```python
from build123d import *

# Parameters (mm, degrees)
SKETCH_W               = 20
SKETCH_H               = 7
PAD_DEPTH              = 7
FILLET_R               = 6.5
MIRROR_ROLL_ANGLE      = -179.860318
MIRROR_PITCH_ANGLE     = 1.669328
MIRROR_PLACEMENT_ANGLE = 0.337481


with BuildPart() as body:
    # Sketch → Pad (new body)
    with BuildSketch(Plane.XY):
        Polygon((0, 290), (50, 290), (150, 0), (120, 0), (120, 13.2), (30, 13.2), (30, 0), (0, 0), align=None)
        Polygon((15, 210), (15, 130), (89.30566, 130), (61.719453, 210), align=None, mode=Mode.SUBTRACT)
        Polygon((15, 110), (15, 33.2), (122.684971, 33.2), (96.202212, 110), align=None, mode=Mode.SUBTRACT)
        Polygon((18, 280), (18, 230), (54.822902, 230), (37.581522, 280), align=None, mode=Mode.SUBTRACT)
        with Locations((28, 220)):
            Rectangle(SKETCH_W, SKETCH_H, mode=Mode.SUBTRACT)
        with Locations((28, 120)):
            Rectangle(SKETCH_W, SKETCH_H, mode=Mode.SUBTRACT)
        with Locations((70.5, 120)):
            Rectangle(SKETCH_W, SKETCH_H, mode=Mode.SUBTRACT)
        with Locations((28, 23.2)):
            Rectangle(SKETCH_W, SKETCH_H, mode=Mode.SUBTRACT)
        with Locations((111, 23.2)):
            Rectangle(SKETCH_W, SKETCH_H, mode=Mode.SUBTRACT)
    extrude(amount=PAD_DEPTH)

    # Fillet
    fillet_edges = [body.edges().sort_by_distance(p)[0] for p in [
        (0, 0, 3.5),
        (50, 290, 3.5),
        (0, 290, 3.5),
        (150, 0, 3.5),
        (120, 0, 3.5),
        (30, 0, 3.5),
        (61.719453, 210, 3.5),
        (15, 210, 3.5),
        (96.202212, 110, 3.5),
        (15, 110, 3.5),
        (15, 130, 3.5),
        (15, 33.2, 3.5),
        (122.684971, 33.2, 3.5),
        (89.30566, 130, 3.5),
        (30, 13.2, 3.5),
        (120, 13.2, 3.5),
        (18, 280, 3.5),
        (18, 230, 3.5),
        (37.581522, 280, 3.5),
        (54.822902, 230, 3.5),
    ]]
    fillet(fillet_edges, radius=FILLET_R)


with BuildPart() as body_1:
    # Body placement: moved
    add(body.part.moved(Location((-2, 0, 0))))


with BuildPart() as body_mirrored:
    # mirror: instance of Body
    add(body_1.part.mirror(Plane(origin=(159.181488, 124.226166, 5.790833), x_dir=(-0.001618, 0.999999, 0), z_dir=(-0.999887, -0.001617, 0.014919))))


with BuildPart() as body_mirrored_1:
    # mirror roll: moved
    add(body_mirrored.part.rotate(Axis((0, 0, 0), (1, 0, 0)), MIRROR_ROLL_ANGLE))


with BuildPart() as body_mirrored_2:
    # mirror pitch: moved
    add(body_mirrored_1.part.rotate(Axis((0, 0, 0), (0, 1, 0)), MIRROR_PITCH_ANGLE))


with BuildPart() as body_mirrored_3:
    # mirror placement: moved
    add(body_mirrored_2.part.moved(Location((-113.201923, 287.892908, 10.586))).rotate(Axis((-113.201923, 287.892908, 10.586), (0, 0, 1)), MIRROR_PLACEMENT_ANGLE))


solid = body_mirrored_3.part
```
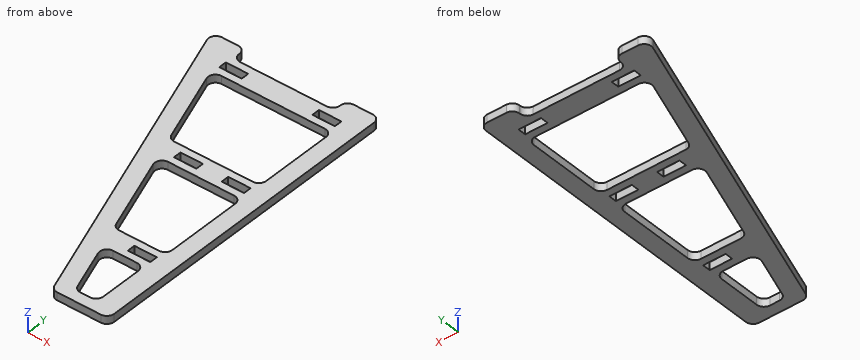
Input: part model. Units: mm. Frame: model coordinates. Give positions to 0.01 mm unless a question says otherwise; leave off trailing zeros. Order: outer loops, then holes, each group sorted by start corner. A loop starts at its lowest first (then second) coordinate and runs counter-clockwise, first axis right, second up.
1. Section B-B on y = 228.5. Return the cut outline in (x, z), and give its area (3 significant figures).
Derived:
outline: (78.31, 5.82) - (78.32, -1.18) - (94.2, -1.17) - (94.19, 5.83) - close; (192.48, -1.1) - (207.48, -1.09) - (207.48, 5.91) - (192.48, 5.9) - close
area: 216 mm2
2. Pin query (flat end, axial travel): pin 1 (1.5 mm diameter, centred on x = 167.5, z = 0, fed in from +Y); pin 2 (1 mm diameter, centred on y = 33, z = 1, fed in from -X); pin 3 (1.5 mm diameter, centred on y = 196.5, z = -1, fed in from -X). Return the tip coordinate at first contact, or that it passes through.
Derived:
pin 1: stops at y = 275.96
pin 2: stops at x = 146.12
pin 3: stops at x = 89.18
3. Section D-D on z = 0.25. Give the number of separate pieces and of enclosed holes in the cut face, and give its area (3 significant figures).
Derived:
separate pieces: 1
enclosed holes: 8
area: 13,700 mm2
4. Section C-C on x = 70.5. Return the cut outline in (y, z).
Derived:
outline: (250.96, 5.87) - (250.99, -1.13) - (288.91, -1.04) - (288.89, 5.96) - close
5. Section A-A on y = 69. Return the cut outline in (x, z).
Derived:
outline: (133.77, 5.48) - (133.78, -1.52) - (169.89, -1.5) - (169.89, 5.5) - close; (189.89, -1.48) - (207.89, -1.47) - (207.89, 5.53) - (189.89, 5.52) - close
6. Material intervals for L1, parallel to Z at x = 199, y = 112.5; L2, parallel to X at y = 138.5, z = 0.5; L3, parallel to X at y = 45.5, z = 4, sorted ascending.
Derived:
L1: z = -1.37 to 5.63
L2: x = 109.61 to 125.49, 192.71 to 207.71
L3: x = 141.94 to 157.82, 189.95 to 207.95
